Verification items for the finished model (mm, model axes). Face numbers are marked on the shaded views. A direction names the side the tool comes from. Round coordinates to 2 decimals unless told otherwise and drop trailing zeros. Write each loop counter-clockwise with the first axis right and the second up, starting at its lowest first coordinate (ties: lowest second). Pieces come first, ordered by that corner, then holes. Notation, with made-up numbers: (-24, 88.5) -> (6, 88.5) arc R37 ccw to (6, 126.5) -> close; hole circle Ø3 at (83.5, 25.25). An arc over 180 degrees is marked (long way). Answer as a JSON object with one key per item and string values. Group by question number.
(1) Set-up check for the marked faces 1 and 2: record each of +Z, -Z, +X, -X, +Y, -Y from which the full face is reachable in a straight line by a thin tool's end or side.
(2) Draft check along X on the marked faces 3, 4 and 5. Enter one of: released by +X, released by -X, zero draft, split by the parting line, or undercut.
(3) Sectioned sample at D-D on y = -16.5. Record the cut outline in (x, z), and give its area (3 significant figures).
(4) Scan lines: L1, parallel to X at y = -21, z = 12.75; L2, parallel to X at y = -10.75, z = 9.25; L3, parallel to X at y = -14.25, z = 21.5. Record each from-to range of solid material in increasing order. Write a range as from..to.
(5) Sectioned sample at B-B on z = 15. Record the cut outline in (x, y) (3 decimals), and give its area (3 significant figures).
(6) Sectioned sample at A-A on z = 21.5. Record the cut outline in (x, y), and give its area (3 significant figures).
(7) Sectioned sample at C-C on x = 30.5. Record the cut outline in (y, z), and give its area (3 significant figures).
(8) Gauge pin test, flat end, axial feed: pin 1 Ø10.5 at (x, y) = (21.5, -5.5) entering from +Z. Record the tip position at first contact, or that the pin passes through.
```python
from build123d import *

# Parameters (mm, degrees)
F1_DEPTH = 22
F3_D     = 8
F5_D     = 8


with BuildPart() as f1:
    # F0 (on Front) → F1 (new body)
    with BuildSketch(Plane.XZ):
        Polygon((0, 25), (0, 0), (40, 0), (40, 25), (26.6667, 25), (26.6667, 20), (13.3337, 20), (13.3337, 25), align=None)
    extrude(amount=F1_DEPTH)

    # F3 (through all)
    with Locations(Plane.XZ.offset(22)):
        with Locations((8.928183, 12.672609)):
            Hole(F3_D / 2)

    # F5 (through all)
    with Locations(Plane.XZ.offset(22)):
        with Locations((30.394303, 12.5)):
            Hole(F5_D / 2)


solid = f1.part
```
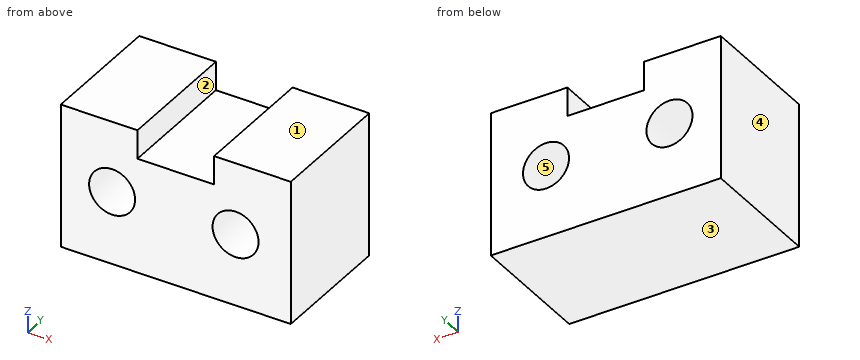
Computed values:
{
 "1": {"face 1": "+Z, +X, -X, +Y, -Y", "face 2": "+Z, +Y, -Y"},
 "2": {"face 3": "zero draft", "face 4": "released by -X", "face 5": "undercut"},
 "3": {"outline": "(0, 0) -> (40, 0) -> (40, 25) -> (26.67, 25) -> (26.67, 20) -> (13.33, 20) -> (13.33, 25) -> (0, 25) -> close; hole circle Ø8 at (8.93, 12.67); hole circle Ø8 at (30.39, 12.5)", "area": "833 mm2"},
 "4": {"L1": "0..4.93, 12.93..26.4, 34.39..40", "L2": "0..6.86, 11..28.06, 32.73..40", "L3": "0..13.33, 26.67..40"},
 "5": {"outline": "(0, -22) -> (5.675, -22) -> (5.675, 0) -> (0, 0) -> close; (12.181, -22) -> (27.272, -22) -> (27.272, 0) -> (12.181, 0) -> close; (33.517, -22) -> (40, -22) -> (40, 0) -> (33.517, 0) -> close", "area": "599 mm2"},
 "6": {"outline": "(0, -22) -> (13.33, -22) -> (13.33, 0) -> (0, 0) -> close; (26.67, -22) -> (40, -22) -> (40, 0) -> (26.67, 0) -> close", "area": "587 mm2"},
 "7": {"outline": "(-22, 0) -> (0, 0) -> (0, 8.5) -> (-22, 8.5) -> close; (-22, 16.5) -> (0, 16.5) -> (0, 25) -> (-22, 25) -> close", "area": "374 mm2"},
 "8": {"pin 1": "z = 25"}
}
